Geometry check sheet. Reference: the model listing, model coordinates, mm. Give positions to 0.01 mm unless a question says otherwise; leave off trailing zeros. Write each loop counter-clockwise with the first axis right and the second up, starting at its lowest first coordinate (ties: lowest second). Pieces come first, ordered by that corner, then holes.
(1) Cross-section at B-B (x = 95.25). Record the boundary of the cut face in (y, z) (3 decimals).
(2) Thickness scan on line 1 along Y through (x, z) = (95.25, 0.6) (3 decimals). Record the ranges inside material, lowest first.
(3) Cross-section at A-A (y = 22.86). Record the boundary of the cut face in (x, z) (3 decimals), and give its area (3 significant figures).
(4) Mould release check, pull along Y, two halves, no side actions. Record for faces 1 (the cylindrical face through (5.94, 21, 0.64)), 2 (the flat face through (50, 23, 0)): +Y half, -Y half, draft (parallel to the pull), parting line (faces both ways), or undercut.
```python
from build123d import *

# Parameters (mm, degrees)
SKETCH1_W          = 101.6
SKETCH1_H          = 45.72
BASE_EXTRUDE_DEPTH = 1.27
HOLE_CUT_REACH     = 113.42
SKETCH2_R          = 1.905


with BuildPart() as part:
    # Sketch1 → Base Extrude (new body)
    with BuildSketch(Plane.XY):
        with Locations((50.8, 22.86)):
            Rectangle(SKETCH1_W, SKETCH1_H)
    extrude(amount=BASE_EXTRUDE_DEPTH)

    # Sketch2 → Hole Cut (cut, up to next)
    with BuildSketch(Plane.XY.offset(1.27), mode=Mode.PRIVATE) as hole_cut_sk1:
        with Locations((6.35, 22.86)):
            Circle(SKETCH2_R)
    hole_cut_tool1 = extrude(hole_cut_sk1.sketch, amount=-HOLE_CUT_REACH, mode=Mode.PRIVATE) & part.part
    # Sketch2 → Hole Cut (cut, up to next)
    with BuildSketch(Plane.XY.offset(1.27), mode=Mode.PRIVATE) as hole_cut_sk2:
        with Locations(Location((95.25, 22.86, 0), (0, 0, 180))):
            Circle(SKETCH2_R)
    hole_cut_tool2 = extrude(hole_cut_sk2.sketch, amount=-HOLE_CUT_REACH, mode=Mode.PRIVATE) & part.part
    add(hole_cut_tool1.solids().sort_by_distance((6.35, 22.86, 1.27))[0], mode=Mode.SUBTRACT)
    add(hole_cut_tool2.solids().sort_by_distance((95.25, 22.86, 1.27))[0], mode=Mode.SUBTRACT)


solid = part.part
```
Reply:
1. outline: (0, 0) - (20.955, 0) - (20.955, 1.27) - (0, 1.27) - close; (24.765, 0) - (45.72, 0) - (45.72, 1.27) - (24.765, 1.27) - close
2. line 1: y = 0 to 20.955, 24.765 to 45.72
3. outline: (0, 0) - (4.445, 0) - (4.445, 1.27) - (0, 1.27) - close; (8.255, 0) - (93.345, 0) - (93.345, 1.27) - (8.255, 1.27) - close; (97.155, 0) - (101.6, 0) - (101.6, 1.27) - (97.155, 1.27) - close
3. area: 119 mm2
4. face 1: undercut
4. face 2: draft
